Read the model definition and answer for the solid it produces. Units are mm, in the model's axes. A direction names the side the tool comes from. Coordinates: 2 decimals unless noted, no trailing zeros. Order: outer loops, then holes, each group sorted by start corner. A loop starts at its lowest first (then second) coordinate and runs counter-clockwise, first axis right, second up. Notation, with made-up numbers: (25, -22) -> (78, -22) arc R20 cw to (78, -13) -> close; hole circle Ø1 at (42, 33). An arc over 180 degrees is marked (long way). Answer as a JSON object with one key per item and string values. Group by question number.
1) Section D-D on x = 6 is taken. Determine the outline of the cut face in (y, z).
2) Section A-A on x = 26 is taken. Determine the outline of the cut face in (y, z).
3) Consider L1, parallel to X at y = 3.25, z = 5; L2, parallel to Y at x = 18, z = 49.4; L3, parallel to Z at x = -26, y = -6.5. Determine where each line is inside the solid, lowest interval first.
4) Section B-B on y = -9.5 is taken. Count the separate pieces of the cut face and the enclosed holes in it, and give its area (3 significant figures).
5) Determine the mould class of faces 1 (the cylindrical face through (28.5, -9.43, 49.51)), 2 (the flat face through (9, 22, 10)), 3 (the cylindrical face through (-28.5, 0.2, 4.9)), 4 (the flat face through (9, 22, 35)) for opening direction Z: released by +Z, released by -Z, zero draft, split by the parting line, or undercut.
6) Given pin 1 (12 mm diameter, centred on y = 23, z = 17.5, fed in from -X); pin 2 (0.9 mm diameter, centred on x = 17.5, y = -9.5, fed in from +Z); pin 3 (1.5 mm diameter, centred on x = -25, y = 16, fed in from +Z); pin 4 (12 mm diameter, centred on x = 3, y = 22.5, fed in from +Z), each flat-ended and moving along its own axis, determine where each tip first touches the part or whether it passes through.
7) A tool of negligible diameter and unlimited length cuts with its end or side. For faces 5 (the flat face through (35, 22, 23)), 6 (the flat face through (-1, 0, 50)), 7 (the flat face through (-30, -9, 49)), from which of +Z, -Z, +X, -X, +Y, -Y can it reach the whole face along a straight path? Write none if from no direction.
8) Section C-C on z = 28.5 is taken. Determine the outline of the cut face in (x, y), and give its area (3 significant figures).
from build123d import *

# Parameters (mm, degrees)
SKETCH1_W               = 72
SKETCH1_H               = 29
BOSS_EXTRUDE1_DEPTH     = 50
SKETCH3_R               = 2.5
SKETCH3_W               = 51
SKETCH3_H               = 25
BOSS_EXTRUDE3_DEPTH     = 15
SKETCH2_R               = 1.5
CUT_EXTRUDE1_DEPTH      = 1
SKETCH4_R               = 2.5
CUT_EXTRUDE2_DEPTH      = 40
CUT_EXTRUDE2_DEPTH_BACK = 40


with BuildPart() as part:
    # Sketch1 → Boss-Extrude1 (new body)
    with BuildSketch(Plane.XY):
        Rectangle(SKETCH1_W, SKETCH1_H)
    extrude(amount=BOSS_EXTRUDE1_DEPTH)

    # Sketch3 → Boss-Extrude3 (add)
    with BuildSketch(Plane(origin=(0, 14.5, 0), x_dir=(1, 0, 0), z_dir=(0, 1, 0))):
        with Locations((-26, -5)):
            Circle(SKETCH3_R)
        with Locations((26, -5)):
            Circle(SKETCH3_R)
        with Locations((9.5, -22.5)):
            Rectangle(SKETCH3_W, SKETCH3_H)
    extrude(amount=BOSS_EXTRUDE3_DEPTH)

    # Sketch2 → Cut-Extrude1 (cut)
    with BuildSketch(Plane.XY.offset(50)):
        with Locations((-30, -9.5)):
            Circle(SKETCH2_R)
        with Locations((-18, -9.5)):
            Circle(SKETCH2_R)
        with Locations((-6, -9.5)):
            Circle(SKETCH2_R)
        with Locations((6, -9.5)):
            Circle(SKETCH2_R)
        with Locations((18, -9.5)):
            Circle(SKETCH2_R)
        with Locations((30, -9.5)):
            Circle(SKETCH2_R)
    extrude(amount=-CUT_EXTRUDE1_DEPTH, mode=Mode.SUBTRACT)

    # Sketch4 → Cut-Extrude2 (cut, two sides)
    with BuildSketch(Plane(origin=(0, 14.5, 0), x_dir=(1, 0, 0), z_dir=(0, 1, 0))) as cut_extrude2_sk:
        with Locations((26, -5)):
            Circle(SKETCH4_R)
        with Locations((-26, -5)):
            Circle(SKETCH4_R)
    extrude(amount=CUT_EXTRUDE2_DEPTH, mode=Mode.SUBTRACT)
    extrude(cut_extrude2_sk.sketch, amount=-CUT_EXTRUDE2_DEPTH_BACK, mode=Mode.SUBTRACT)


solid = part.part
Worked answers:
{
 "1": {"outline": "(-14.5, 0) -> (14.5, 0) -> (14.5, 10) -> (29.5, 10) -> (29.5, 35) -> (14.5, 35) -> (14.5, 50) -> (-8, 50) -> (-8, 49) -> (-11, 49) -> (-11, 50) -> (-14.5, 50) -> close"},
 "2": {"outline": "(-14.5, 0) -> (14.5, 0) -> (14.5, 2.5) -> (-14.5, 2.5) -> close; (-14.5, 7.5) -> (14.5, 7.5) -> (14.5, 10) -> (29.5, 10) -> (29.5, 35) -> (14.5, 35) -> (14.5, 50) -> (-14.5, 50) -> close"},
 "3": {"L1": "x = -36 to -28.5, -23.5 to 23.5, 28.5 to 36", "L2": "y = -14.5 to -11, -8 to 14.5", "L3": "z = 0 to 2.5, 7.5 to 50"},
 "4": {"separate pieces": "1", "enclosed holes": "2", "area": "3,540 mm²"},
 "5": {"face 1": "zero draft", "face 2": "released by -Z", "face 3": "undercut", "face 4": "released by +Z"},
 "6": {"pin 1": "stops at x = -16", "pin 2": "stops at z = 49", "pin 3": "passes through", "pin 4": "stops at z = 35"},
 "7": {"face 5": "+Z, -Z, +X, +Y", "face 6": "+Z, +X, -X, +Y, -Y", "face 7": "+Z"},
 "8": {"outline": "(-36, -14.5) -> (36, -14.5) -> (36, 14.5) -> (35, 14.5) -> (35, 29.5) -> (-16, 29.5) -> (-16, 14.5) -> (-36, 14.5) -> close", "area": "2,850 mm²"}
}
